Work out the finished part from the listing and answer in its coordinate system (mm). Coordinates: 2 decimals unless noted, no trailing zeros. Order: outer loops, then holes, each group sorted by start corner. A loop starts at its lowest first (then second) coordinate and runs counter-clockwise, first axis right, second up. Notation, with made-up numbers: M 46.25,8 L 54.25,8 A11 cw 54.25,18 Z; hole C -27.5,31.25 d8. An arc over 180 degrees is marked long. Use a Markdown table: item, result.
from build123d import *

# Parameters (mm, degrees)
EXTRUDE_2_DEPTH     = 76
SKETCH_5_W          = 69.282032302
SKETCH_5_H          = 17
CUT_EXTRUDE_2_DEPTH = 51
SKETCH_7_W          = 79.816599869
SKETCH_7_H          = 73.41094556
CUT_EXTRUDE_3_DEPTH = 51


with BuildPart() as part:
    # 草图1 → 凸台-拉伸2 (new body)
    with BuildSketch(Plane(origin=(0, 0, 0), x_dir=(1, 0, 0), z_dir=(0, 1, 0))):
        Polygon((0, 34.641016151), (-30, 17.320508076), (-30, -17.320508076), (0, -34.641016151), (30, -17.320508076), (30, 17.320508076), align=None)
    extrude(amount=EXTRUDE_2_DEPTH)

    # 草图5 → 切除-拉伸2 (cut)
    with BuildSketch(Plane(origin=(30, 0, 0), x_dir=(0, 0, -1), z_dir=(1, 0, 0))):
        with Locations((0, 67.5)):
            Rectangle(SKETCH_5_W, SKETCH_5_H)
    extrude(amount=-CUT_EXTRUDE_2_DEPTH, mode=Mode.SUBTRACT)

    # 草图7 → 切除-拉伸3 (cut)
    with BuildSketch(Plane(origin=(20.8024046, 30.312075274, 0), x_dir=(-0.824513353, 0.565842497, 0), z_dir=(-0.565842497, -0.824513353, 0))):
        with Locations((10.791187789, -0.103687776)):
            Rectangle(SKETCH_7_W, SKETCH_7_H)
    extrude(amount=-CUT_EXTRUDE_3_DEPTH, mode=Mode.SUBTRACT)


solid = part.part
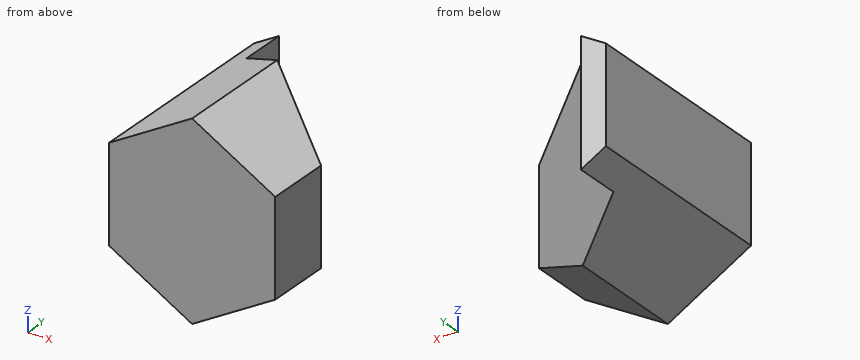
1. Section A-A on y = 65 is taken. Determine the outline of the cut face in (x, z).
Answers below:
| item | result |
|---|---|
| outline | M -30,-17.32 L -21,-22.52 L -21,22.52 L -30,17.32 Z |
2. Flat-ended cylindrical pins translate along their axes: P1, Ø5, axis at y = 59.5, z = 8.5, coming from the +X side; P2, Ø1, axis at x = 5.5, z = -5.5, coming from the +Y side; P3, Ø1.5, axis at y = 65.5, z = 16, coming from the +X side. Find the tip coordinate at first contact, or state that the pin passes through.
Answers below:
| item | result |
|---|---|
| P1 | x = -18.09 |
| P2 | y = 41.16 |
| P3 | x = -21 |
3. Section C-C on x = 5 is taken. Determine the outline of the cut face in (y, z).
Answers below:
| item | result |
|---|---|
| outline | M 0,-31.75 L 41.16,-31.75 L 41.16,31.75 L 0,31.75 Z |
4. Find the intervals of material crossed by probe 1 along Y at (x, z) = (0, 0); probe 2 along X at (y, z) = (72, 4.5); probe 3 along X at (y, z) = (35.5, -12.5), in increasing order.
Answers below:
| item | result |
|---|---|
| probe 1 | 0 to 44.59 |
| probe 2 | -30 to -21 |
| probe 3 | -30 to 13.24 |
5. Section D-D on y = 34 is taken. Determine the outline of the cut face in (x, z), then the cut area to 3 significant figures.
Answers below:
| item | result |
|---|---|
| outline | M -30,-17.32 L 0,-34.64 L 15.43,-25.73 L 15.43,25.73 L 0,34.64 L -30,17.32 Z |
| area | 2,490 mm² |
6. Section B-B on z = -13.5 is taken. Determine the outline of the cut face in (x, y).
Answers below:
| item | result |
|---|---|
| outline | M -30,0 L 30,0 L 30,24 L -21,59 L -21,76 L -30,76 Z |
